Autodesk Inventor part; units mm, degrees
ref_plane "YZ Plane" through (0, 0, 0) normal (1, 0, 0) x (0, 1, 0)
ref_plane "XZ Plane" through (0, 0, 0) normal (0, 1, 0) x (-1, 0, 0)
ref_plane "XY Plane" through (0, 0, 0) normal (0, 0, 1) x (1, 0, 0)
sketch "스케치1" plane through (0, 0, 0) normal (0, 0, 1) x (1, 0, 0)
  circle A0 centre (0, 0) radius 30
  dimension "d0" = 60
extrude "돌출1" add sketch "스케치1" along normal blind 8
sketch "스케치2" plane through (0, 0, 8) normal (0, 0, 1) x (1, 0, 0)
  circle A0 centre (0, 0) radius 17.5
  dimension "d3" = 35
extrude "돌출2" add sketch "스케치2" along normal blind 4
sketch "스케치3" plane through (0, 0, 0) normal (0, 0, -1) x (-1, 0, 0)
  circle A0 centre (0, 0) radius 16
  dimension "d6" = 32
extrude "돌출3" add sketch "스케치3" along normal blind 4
sketch "스케치4" plane through (0, 0, 12) normal (0, 0, 1) x (1, 0, 0)
  circle A0 centre (0, 0) radius 15
  dimension "d9" = 30
extrude "돌출4" cut sketch "스케치4" against normal blind 5
sketch "스케치5" plane through (0, 0, 7) normal (0, 0, 1) x (1, 0, 0)
  circle A0 centre (0, 0) radius 7
  dimension "d12" = 14
extrude "돌출5" cut sketch "스케치5" against normal blind 8
sketch "스케치6" plane through (0, 0, -1) normal (0, 0, 1) x (1, 0, 0)
  circle A0 centre (0, 0) radius 12.5
  dimension "d15" = 25
extrude "돌출6" cut sketch "스케치6" against normal up to next
sketch "스케치7" plane through (0, 0, 0) normal (0, 0, -1) x (-1, 0, 0)
  circle A0 centre (0, 23) radius 2.25
  point P0 (0, 0)
  dimension "d18" = 4.5
  dimension "d19" = 23
hole "구멍1" at (0, 23, 0) direction (0, 0, 1) diameter 4.5 end through all counterbore diameter 8 counterbore depth 4.4
pattern_circular "원형 패턴1" count 3 over 360 about axis through (0, 0, 0) along (0, 0, 1) of "구멍1"
chamfer "모따기1" distance 0.4 angle 30 1 edges at (-12.5, 0, -4) measured on face at (12.4595, -1.0058, -3)
fillet "모깎기1" radius 0.5 1 edges at (-12.5, 0, -1)
chamfer "모따기2" distance 1 angle 45 1 edges at (-17.5, 0, 12)
fillet "모깎기2" radius 3 4 edges at (-30, 0, 0) (16, 0, 0) (16, 0, -4) (-15, 0, 7)
properties part number "2강2"
The model under review builds one solid part; all positions refer to its coordinate system, in mm. A direction names the side the tool comes from. Coordinates: 2 decimals unless noted, no trailing zeros.
(1) Wall thickness on L1, parallel to X at y = -11.5, z = 5.3; L2, parallel to X at y = -11.5, z = 1.5; L3, parallel to Y at x = -3, z = 3.75: over which ranges is each line inside the solid? List them lowest first.
Determined:
L1: x = -27.71 to -22.17, -17.67 to 17.67, 22.17 to 27.71
L2: x = -27.27 to -23.92, -15.92 to 15.92, 23.92 to 27.27
L3: y = -29.85 to -6.32, 6.32 to 20.35, 25.65 to 29.85
(2) Draft analysis for pull direction X (two halves, no side actions). For faces 1 (the flat face through (4, -15, 12)), 2 (the flat face through (5.2, -5.2, 7)), 3 (the cylindrical face through (-29.97, -1.32, 5.46)), state which applies: +X half, -X half, draft (parallel to the pull), parting line (faces both ways), or undercut.
Determined:
face 1: draft
face 2: undercut
face 3: parting line
(3) Insertion check: P1, Ø4, axis at x = 20, y = -12, coming from the -Z side; P2, Ø5, axis at x = 0, y = 23, coming from the +Z side; P3, Ø6.5, axis at x = 0, y = 24, coming from the -Z side. Each pin has a flat end and moves straight along its axis. Give the tip position at first contact, or say it passes through.
Determined:
P1: stops at z = 4.4
P2: stops at z = 8
P3: stops at z = 0
(4) Tool access review of faces 4 (the cylindrical face through (-0.676, 25.146, 6.225)), 5 (the cylindrical face through (-14.985, 0.66, 11.014)), 6 (the cylindrical face through (16.546, -9.35, 2.231)): name each direction out of +Z, -Z, +X, -X, +Y, -Y from which nothing blocks a thin tool from reaching the whole face with its end or side.
Determined:
face 4: +Z, -Z
face 5: +Z
face 6: -Z
(5) Consider section A-A, the plane x = 0. Give the number of separate pieces and of enclosed holes in the cut face, plus the area to 3 significant figures.
Determined:
separate pieces: 3
enclosed holes: 0
area: 360 mm2
